```python
from build123d import *

# Parameters (mm, degrees)
SKETCH1_R           = 2.5
SKETCH1_R_2         = 1.5
BOSS_EXTRUDE1_DEPTH = 6.3
SKETCH2_R           = 3.25
CUT_EXTRUDE1_DEPTH  = 4.5
CHAMFER1_SIZE       = 0.5


with BuildPart() as part:
    # Sketch1 → Boss-Extrude1 (new body)
    with BuildSketch(Plane(origin=(0, 0, 0), x_dir=(1, 0, 0), z_dir=(0, 1, 0))):
        with BuildLine():
            Line((40, 15), (-40, 15))
            ThreePointArc((-40, 15), (-47.071067812, 12.071067812), (-50, 5))
            Line((-50, 5), (-50, -5))
            ThreePointArc((-50, -5), (-47.071067812, -12.071067812), (-40, -15))
            Line((-40, -15), (40, -15))
            ThreePointArc((40, -15), (47.071067812, -12.071067812), (50, -5))
            Line((50, -5), (50, 5))
            ThreePointArc((50, 5), (47.071067812, 12.071067812), (40, 15))
        make_face()
        with Locations(Location((43, 0, 0), (0, 0, 270))):
            Circle(SKETCH1_R, mode=Mode.SUBTRACT)
        with Locations(Location((-43, 0, 0), (0, 0, 90))):
            Circle(SKETCH1_R, mode=Mode.SUBTRACT)
        with Locations(Location((0, -9.5, 0), (0, 0, 270))):
            Circle(SKETCH1_R_2, mode=Mode.SUBTRACT)
        with Locations(Location((-9.5, 0, 0), (0, 0, 270))):
            Circle(SKETCH1_R_2, mode=Mode.SUBTRACT)
        with Locations(Location((0, 9.5, 0), (0, 0, 270))):
            Circle(SKETCH1_R_2, mode=Mode.SUBTRACT)
        with Locations(Location((9.5, 0, 0), (0, 0, 270))):
            Circle(SKETCH1_R_2, mode=Mode.SUBTRACT)
    extrude(amount=BOSS_EXTRUDE1_DEPTH)

    # Sketch2 → Cut-Extrude1 (cut)
    with BuildSketch(Plane.XZ):
        with Locations(Location((0, 9.5, 0), (0, 0, 270))):
            Circle(SKETCH2_R)
        with Locations(Location((9.5, 0, 0), (0, 0, 270))):
            Circle(SKETCH2_R)
        with Locations(Location((0, -9.5, 0), (0, 0, 270))):
            Circle(SKETCH2_R)
        with Locations(Location((-9.5, 0, 0), (0, 0, 270))):
            Circle(SKETCH2_R)
    extrude(amount=-CUT_EXTRUDE1_DEPTH, mode=Mode.SUBTRACT)

    # Chamfer1
    chamfer1_edges = [part.edges().sort_by_distance(p)[0] for p in [
        (0, 0, 15),
        (-47.071067812, 0, 12.071067812),
        (-50, 0, 0),
        (-47.071067812, 0, -12.071067812),
        (-47.071067812, 6.3, 12.071067812),
        (0, 6.3, 15),
        (47.071067812, 6.3, 12.071067812),
        (43, 0, -2.5),
        (43, 6.3, -2.5),
        (50, 6.3, 0),
        (-43, 0, 2.5),
        (-43, 6.3, 2.5),
        (47.071067812, 6.3, -12.071067812),
        (0, 6.3, 8),
        (0, 6.3, -15),
        (-9.5, 6.3, -1.5),
        (0, 6.3, -11),
        (9.5, 6.3, -1.5),
        (-47.071067812, 6.3, -12.071067812),
        (0, 0, 12.75),
        (9.5, 0, 3.25),
        (0, 0, -6.25),
        (-9.5, 0, 3.25),
        (0, 0, -15),
        (-50, 6.3, 0),
        (47.071067812, 0, -12.071067812),
        (50, 0, 0),
        (47.071067812, 0, 12.071067812),
    ]]
    chamfer(chamfer1_edges, length=CHAMFER1_SIZE)


solid = part.part
```
Model file for the job. Use its own axes, mm. A direction names the side the tool comes from. Give positions to 0.01 mm unless a question says otherwise; leave off trailing zeros. Use a Markdown table: item, result.
1) Tool access for faces 1 (the flat face through (50, 3, 0)), 2 (the cylindrical face through (0.143, 2.472, -6.253)): list every direction of +Z, -Z, +X, -X, +Y, -Y with a clear straight run to the whole face (end or side of a thin tool).
Responses:
| item | result |
|---|---|
| face 1 | +Z, -Z, +X, +Y, -Y |
| face 2 | -Y |
2) Pin check, flat tips, straight feed: pin 1 (5 mm diameter, centred on x = 1, z = -10, fed in from -Y); pin 2 (4 mm diameter, centred on x = 0, z = 9.5, fed in from -Y); pin 3 (3.5 mm diameter, centred on x = -9.5, z = 0, fed in from +Y). Stop position of each tip, or through.
Responses:
| item | result |
|---|---|
| pin 1 | stops at y = 0.13 |
| pin 2 | stops at y = 4.5 |
| pin 3 | stops at y = 6.05 |
3) Pull direction Z, two halves, no side cores. Call faces 3 (the flat face through (-1, 4.5, -11)), 4 (the cylindrical face through (-46.99, 3.11, -12.15)), 5 (the cylindrical face through (0.143, 2.472, 12.747)), 6 (the cylindrical face through (-47.15, 3.11, 11.99)): +Z half, -Z half, draft (parallel to the pull), parting line (faces both ways), or undercut.
Responses:
| item | result |
|---|---|
| face 3 | undercut |
| face 4 | -Z half |
| face 5 | undercut |
| face 6 | +Z half |
4) Drill centre lines: line 1 (Z direction, x = 0, y = 5.55); line 2 (X direction, y = 5.25, z = 0); line 3 (X direction, y = 3.5, z = 0). Where is each one in solid material? Low to high. Write a range as from..to.
Responses:
| item | result |
|---|---|
| line 1 | z = -15..-11, -8..8, 11..15 |
| line 2 | x = -50..-45.5, -40.5..-11, -8..8, 11..40.5, 45.5..50 |
| line 3 | x = -50..-45.5, -40.5..-12.75, -6.25..6.25, 12.75..40.5, 45.5..50 |
5) Cut at A-A (x = 0). Give the number of separate pieces and of enclosed holes in the cut face, and give its area (3 significant figures).
Responses:
| item | result |
|---|---|
| separate pieces | 3 |
| enclosed holes | 0 |
| area | 118 mm2 |
